Build history of the part. All positions in model axes, mm. Face numbers are marked on the shaded views. A direction names the side the tool comes from. Round coordinates to 2 decimals unless told otherwise and drop trailing zeros. Write each loop counter-clockwise with the first axis right and the second up, starting at its lowest first coordinate (ties: lowest second). Pieces come first, ordered by that corner, then holes. Notation, with made-up numbers: (34.5, 84) -> (39.5, 84) arc R20 cw to (39.5, 102) -> close; hole circle Ø4 at (9.25, 38). An arc over 180 degrees is marked (long way). Return JSON: item names as keys, results as strings.
from build123d import *

# Parameters (mm, degrees)
BASPROSKE_W          = 19.05
BASPROSKE_H          = 8.89
TOOTHCUT_DEPTH       = 23.82469496
TEETHCUTS_COUNT      = 12
TEETHCUTS_ANGLE      = 330
BORSKE_R             = 1.5875
BORE_DEPTH           = 50.8015748
CUT_EXTRUDE1_START   = -19.05
SKETCH1_R            = 3
CUT_EXTRUDE1_DEPTH   = 3.4798
M3_CLEARANCE_HOLE1_D = 3.4


with BuildPart() as part:
    # BasProSke → Base-Revolve (revolve)
    with BuildSketch(Plane(origin=(0, 0, 0), x_dir=(1, 0, 0), z_dir=(0, 1, 0)), mode=Mode.PRIVATE) as base_revolve_sk:
        with Locations((9.525, 4.445)):
            Rectangle(BASPROSKE_W, BASPROSKE_H)
    revolve(base_revolve_sk.sketch.rotate(Axis((-10, 0, 0), (1, 0, 0)), 180), axis=Axis((-10, 0, 0), (1, 0, 0)))

    # TooCutSke → ToothCut (cut, through all)
    with BuildSketch(Plane(origin=(0, 0, 0), x_dir=(0, 0, -1), z_dir=(1, 0, 0))):
        with BuildLine():
            ThreePointArc((0.717076553, 6.002519826), (0, 6.0452), (-0.717076553, 6.002519826))
            ThreePointArc((-0.717076553, 6.002519826), (-1.069160545, 7.516029346), (-2.121611652, 8.659279483))
            ThreePointArc((-2.121611652, 8.659279483), (0, 8.9154), (2.121611652, 8.659279483))
            ThreePointArc((2.121611652, 8.659279483), (1.069160545, 7.516029346), (0.717076553, 6.002519826))
        make_face()
    toothcut = extrude(amount=TOOTHCUT_DEPTH, mode=Mode.SUBTRACT)

    # TeethCuts: ToothCut ×12 about axis
    teethcuts_axis = Axis((-10, 0, 0), (1, 0, 0))
    for i in range(1, TEETHCUTS_COUNT):
        add(toothcut.rotate(teethcuts_axis, i * TEETHCUTS_ANGLE / (TEETHCUTS_COUNT - 1)), mode=Mode.SUBTRACT)

    # BorSke → Bore (cut, symmetric)
    with BuildSketch(Plane(origin=(0, 0, 0), x_dir=(0, 0, -1), z_dir=(1, 0, 0))):
        with Locations(Location((0, 0, 0), (0, 0, 180))):
            Circle(BORSKE_R)
    extrude(amount=BORE_DEPTH, both=True, mode=Mode.SUBTRACT)

    # Sketch1 → Cut-Extrude1 (cut)
    with BuildSketch(Plane.ZY.offset(CUT_EXTRUDE1_START)):
        Circle(SKETCH1_R)
    extrude(amount=CUT_EXTRUDE1_DEPTH, mode=Mode.SUBTRACT)

    # M3 Clearance Hole1 (through all)
    with Locations(Plane(origin=(0, 0, 0), x_dir=(0, 0, -1), z_dir=(-1, 0, 0))):
        with Locations((0, 0)):
            Hole(M3_CLEARANCE_HOLE1_D / 2)


solid = part.part
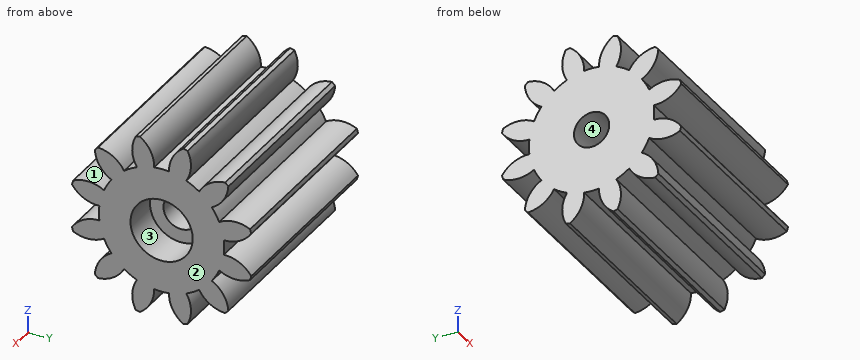
Q1. Saw through at A-A on z = 0. List the corners of the cut face in (x, y), then the cut area to 3 significant figures.
Verdict:
{"outline": "(0, -6.05) -> (19.05, -6.05) -> (19.05, -3) -> (15.57, -3) -> (15.57, -1.7) -> (0, -1.7) -> close; (0, 1.7) -> (15.57, 1.7) -> (15.57, 3) -> (19.05, 3) -> (19.05, 6.05) -> (0, 6.05) -> close", "area": "157 mm²"}
Q2. Two-plate mould, pull along Z, no slides. Class the marked faces 1 and 2: +Z half, -Z half, draft (parallel to the pull), parting line (faces both ways), or undercut.
Verdict:
{"face 1": "undercut", "face 2": "draft"}
Q3. Saw through at C-C on y = 4.5. List the corners of the cut face in (x, z).
Verdict:
{"outline": "(0, -5.85) -> (19.05, -5.85) -> (19.05, 5.85) -> (0, 5.85) -> close"}
Q4. 3-axis set-ups, long thin cutter, end or side, ignore diameter. For the marked faces 3 and 4: which of +Z, -Z, +X, -X, +Y, -Y reach the whole face in a straight line?
Verdict:
{"face 3": "+X", "face 4": "+X, -X"}
Q5. Pin check, flat tips, straight feed: pin 1 Ø3 at (x, z) = (11, 5.5) entering from -Y; pin 2 Ø6 at (x, y) = (13.5, 0.5) entering from +Z; pin 3 Ø1.5 at (x, z) = (8.5, 3) entering from -Y; pin 4 Ø1 at (y, z) = (0.5, 1) entering from +X. Stop position of each tip, or through.
Verdict:
{"pin 1": "stops at y = -6.44", "pin 2": "stops at z = 8.64", "pin 3": "stops at y = -8.6", "pin 4": "passes through"}
Q6. Wall check: L1, parallel to Z at x = 1, y = -8; L2, parallel to Z at x = 7.5, y = 1; L3, parallel to Y at x = 8, z = 6.5. Give the ranges that are in metal, low to high.
Verdict:
{"L1": "z = -2.72 to -1.39, 1.39 to 2.72", "L2": "z = -7.38 to -1.37, 1.37 to 7.38", "L3": "y = -2.76 to -0.74, 0.74 to 2.76"}
